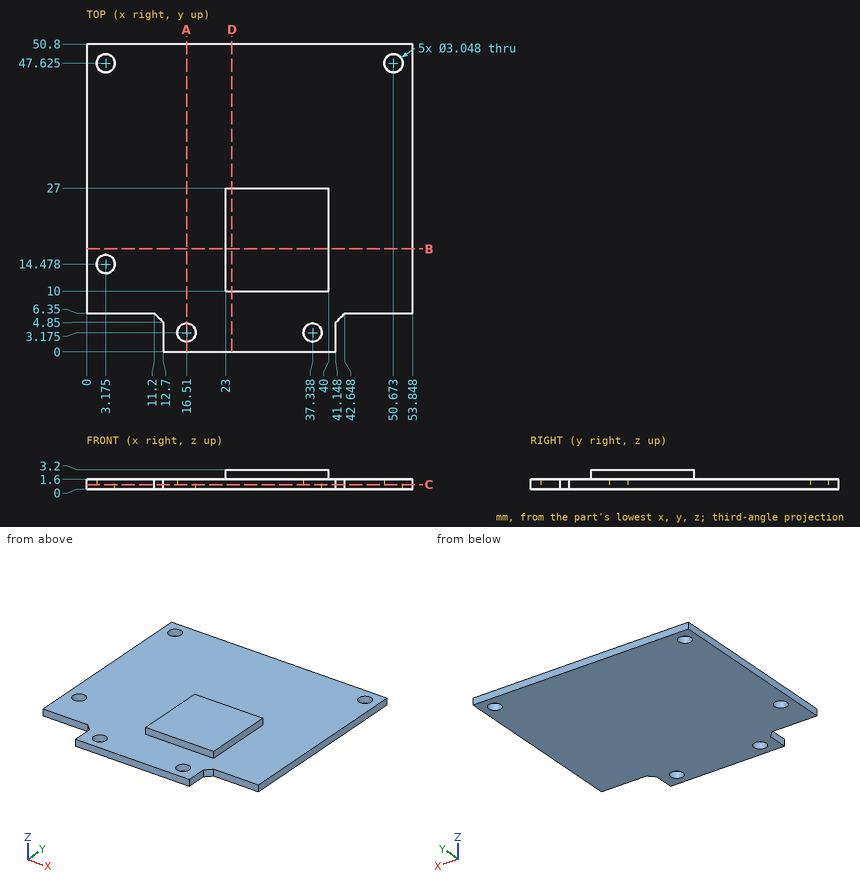
Could you check a few things on this drawing? It's one solid part, dimensions in mm from its lowest x, y, z. Round coordinates to 2 decimals unless told otherwise and drop trailing zeros. Write each loop counter-clockwise with the first axis right and the second up, starting at its lowest first coordinate (ties: lowest second). Pieces come first, ordered by that corner, then holes. Notation, with made-up numbers: (46.25, -10) -> (98.25, -10) arc R26 ccw to (98.25, 10) -> close; hole circle Ø5 at (-2, -35). An arc over 180 degrees is marked (long way). One line per question, with ' | ' between items. Start each with the question number.
1) I need wall thicknesses on line 1 (X direction, y = 47.5, z = 1.3); line 2 (Y direction, x = 16.51, z = 0.95); line 3 (Z direction, x = 13.5, y = 3.5). Which ranges of each line are inside material? Lowest first, please. Write a range as [from, to].
2) Suppose I cut it at C-C on z = 0.75. Write out the boundary of the cut face in (x, y) (3 decimals), then the cut area to 3 significant figures.
3) Suppose I cut it at A-A on x = 16.51. Write out the boundary of the cut face in (y, z).
4) Suppose I cut it at D-D on x = 24. Write out the boundary of the cut face in (y, z).
5) Suppose I cut it at B-B on y = 17. Write out the boundary of the cut face in (x, z), then the cut area to 3 significant figures.
6) I'm going to push flat-ended pins straight in: P1, Ø0.8, axis at y = 1.5, z = 0.5, coming from the +X side; P2, Ø0.8, axis at x = 31.5, z = 2.5, coming from the +Y side; P3, Ø1.3, axis at y = 22.5, z = 2.5, coming from the -X side; P4, Ø3.5, axis at x = 50.673, y = 47.625, coming from the -Z side. Where does each tip first touch, or does it pass through?
Return value:
1) line 1: x = [0, 1.66], [4.69, 49.15], [52.19, 53.85] | line 2: y = [0, 1.65], [4.7, 50.8] | line 3: z = [0, 1.6]
2) outline: (0, 6.35) -> (11.2, 6.35) -> (12.7, 4.85) -> (12.7, 0) -> (41.148, 0) -> (41.148, 4.85) -> (42.648, 6.35) -> (53.848, 6.35) -> (53.848, 50.8) -> (0, 50.8) -> close; hole circle Ø3.048 at (3.175, 14.478); hole circle Ø3.048 at (3.175, 47.625); hole circle Ø3.048 at (16.51, 3.175); hole circle Ø3.048 at (37.338, 3.175); hole circle Ø3.048 at (50.673, 47.625) | area: 2,540 mm2
3) outline: (0, 0) -> (1.65, 0) -> (1.65, 1.6) -> (0, 1.6) -> close; (4.7, 0) -> (50.8, 0) -> (50.8, 1.6) -> (4.7, 1.6) -> close
4) outline: (0, 0) -> (50.8, 0) -> (50.8, 1.6) -> (27, 1.6) -> (27, 3.2) -> (10, 3.2) -> (10, 1.6) -> (0, 1.6) -> close
5) outline: (0, 0) -> (53.85, 0) -> (53.85, 1.6) -> (40, 1.6) -> (40, 3.2) -> (23, 3.2) -> (23, 1.6) -> (0, 1.6) -> close | area: 113 mm2
6) P1: stops at x = 41.15 | P2: stops at y = 27 | P3: stops at x = 23 | P4: stops at z = 0
